Could you check a few things on this model? Use its own coordinates, in mm. Face numbers are marked on the shaded views. Round coordinates to 2 decimals unless told otherwise and drop trailing zeros. Loops run counter-clockwise (first coordinate to the right, second up) from the corner with the lowest first, then second, coordinate; pieces in that order, holes last. Notation, with made-up numbers: (13.25, 85.25) -> (68.25, 85.25) arc R10 cw to (68.25, 93.25) -> close; hole circle Ø11 at (1, -37.5). An arc over 180 degrees is marked (long way). Put each result on its own line as item: value. Start each with the question number.
1. Imagine slicing it at D-D, the plane z = -16.5. Please give me the cut outline in (x, y), and give its area (3 significant figures).
2. Imagine slicing it at A-A, the plane x = 36.5. Please give me the cut outline in (y, z), and give its area (3 significant figures).
3. Imagine slicing it at B-B, the plane y = 0. Please give me the cut outline in (x, z).
4. I'm going to push a flat-ended pin straight in: P1, Ø1, axis at x = 10.5, z = 17, coming from the +Y side. Where does the tip first touch, or does it pass through?
5. I need wall thicknesses on line 1 (Y direction, x = 11.5, z = 0); line 2 (Y direction, x = 3.5, z = 2.5). Which ranges of each line are inside material? Lowest first, please. Write a range as [from, to].
6. If we mould it in two halves opening along Z, with no side actions, what happens to the marked faces 1, 2 and 3? For each: pulls with the +Z half, pulls with the -Z half, needs draft (parallel to the pull), parting line crosses it, or undercut.
```python
from build123d import *

# Parameters (mm, degrees)
PAD_DEPTH       = 46
SKETCH003_R     = 3.5
POCKET001_DEPTH = 46.001
FILLET003_R     = 2


with BuildPart() as part:
    # Sketch002 → Pad (new body)
    with BuildSketch(Plane.YZ):
        Polygon((-21, 14), (-14, 21), (14, 21), (21, 14), (21, -14), (14, -21), (-14, -21), (-21, -14), align=None)
    extrude(amount=PAD_DEPTH)

    # Sketch003 (on Face9 of Pad) → Pocket001 (cut, through all)
    with BuildSketch(Plane(origin=(0, 0, 0), x_dir=(0, 1, 0), z_dir=(-1, 0, 0))):
        Circle(SKETCH003_R)
    extrude(amount=-POCKET001_DEPTH, mode=Mode.SUBTRACT)

    # Fillet003
    fillet003_edges = [part.edges().sort_by_distance(p)[0] for p in [
        (23, -21, -14),
        (23, -21, 14),
        (23, -14, 21),
        (23, 14, 21),
        (23, -14, -21),
        (23, 14, -21),
        (23, 21, -14),
        (23, 21, 14),
    ]]
    fillet(fillet003_edges, radius=FILLET003_R)


solid = part.part
```
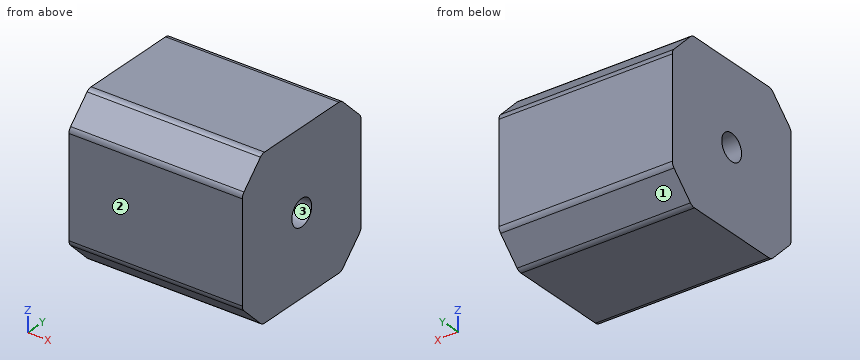
Entries:
1. outline: (0, -18.5) -> (46, -18.5) -> (46, 18.5) -> (0, 18.5) -> close
1. area: 1,700 mm^2
2. outline: (-21, -13.17) arc R2 ccw to (-20.41, -14.59) -> (-14.59, -20.41) arc R2 ccw to (-13.17, -21) -> (13.17, -21) arc R2 ccw to (14.59, -20.41) -> (20.41, -14.59) arc R2 ccw to (21, -13.17) -> (21, 13.17) arc R2 ccw to (20.41, 14.59) -> (14.59, 20.41) arc R2 ccw to (13.17, 21) -> (-13.17, 21) arc R2 ccw to (-14.59, 20.41) -> (-20.41, 14.59) arc R2 ccw to (-21, 13.17) -> close; hole circle Ø7 at (0, 0)
2. area: 1,630 mm^2
3. outline: (0, -21) -> (46, -21) -> (46, -3.5) -> (0, -3.5) -> close; (0, 3.5) -> (46, 3.5) -> (46, 21) -> (0, 21) -> close
4. P1: y = 18.5
5. line 1: [-21, -3.5], [3.5, 21]
5. line 2: [-21, -2.45], [2.45, 21]
6. face 1: pulls with the -Z half
6. face 2: needs draft
6. face 3: undercut
